Study the drawing (mm; zero at the part's minimum x, y, z) and answer. Coordinates: 2 decimals unless noted, no trailing zeros. Write each loop counter-clockwise with the first axis right and the second up, starting at its lowest first coordinate (ties: lowest second). Pieces come first, ordered by that corner, then holes. Notation, with made-up numbers: (-15, -35.5) -> (2, -35.5) arc R12 ccw to (2, -12.5) -> close; hole circle Ø5 at (40, -3.75). An arc over 180 degrees is marked (long way). Write item = value, one per line. Start each with the question number.
1) Flat-ended cylindrical pins translate along their axes: pin 1 Ø12 at (x, y) = (17.5, 14.5) entering from -Z; pin 2 Ø1.5 at (x, z) = (31, 66) entering from -Y; pin 3 Ø1.5 at (x, z) = (18, 37) entering from +Y. Find the tip coordinate at first contact, or state that the pin passes through.
2) Section A-A (y = 5) is taken. Determine the outline of the cut face in (x, z), plus the area to 3 significant figures.
3) For a pull along X with two mould halves and no side action, classify the marked faces 1, 2 and 3 as released by +X, released by -X, zero draft, split by the parting line, or undercut.
4) Section D-D (y = 39) is taken. Determine the outline of the cut face in (x, z) (1 decimal), plus the area to 3 significant figures.
5) Section C-C (z = 73) is taken. Determine the outline of the cut face in (x, y), plus the area to 3 significant figures.
6) Find the intervals of material crossed by line 1 along Z through (x, y) = (28.5, 9.5); line 2 along Y through (x, z) = (24, 76.5); line 3 along X through (y, z) = (20.5, 3), in increasing order. Write a range as from..to.
7) Section B-B (x = 10.5) is taken. Determine the outline of the cut face in (y, z) (1 decimal).
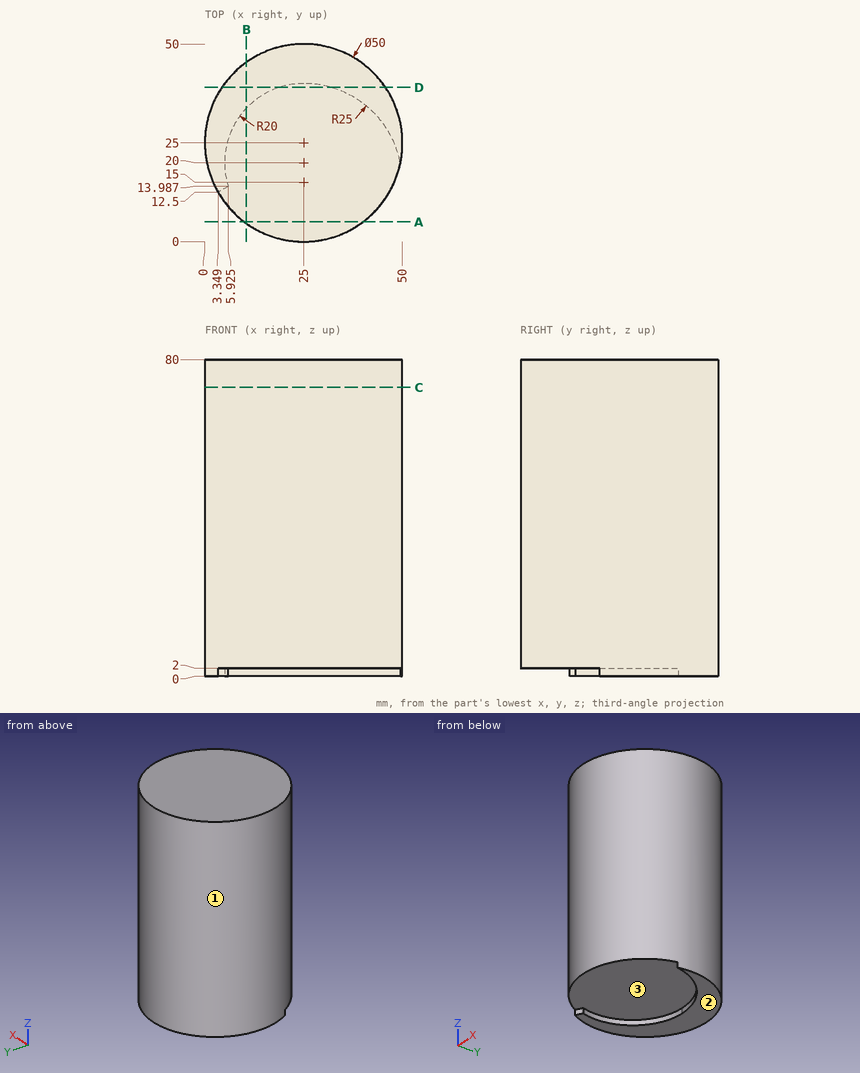
Answer key:
q1.pin_1 = 2
q1.pin_2 = 0.56
q1.pin_3 = 49.21
q2.outline = (10, 2) -> (40, 2) -> (40, 80) -> (10, 80) -> close
q2.area = 2,340 mm^2
q3.face_1 = split by the parting line
q3.face_2 = zero draft
q3.face_3 = undercut
q4.outline = (4.3, 0) -> (18.8, 0) -> (18.8, 2) -> (32, 2) -> (32, 0) -> (45.7, 0) -> (45.7, 80) -> (4.3, 80) -> close
q4.area = 3,290 mm^2
q5.outline = circle Ø50 at (25, 25)
q5.area = 1,960 mm^2
q6.line_1 = 2..80
q6.line_2 = 0.02..49.98
q6.line_3 = 0.41..49.59
q7.outline = (4.6, 2) -> (33.8, 2) -> (33.8, 0) -> (45.4, 0) -> (45.4, 80) -> (4.6, 80) -> close
